from build123d import *

# Parameters (mm, degrees)
F0_W      = 24
F0_H      = 24
F0_R      = 2.6
F1_DEPTH  = 24
F2_SIZE   = 2
F4_DEPTH  = 8
F5_R      = 2
F7_DEPTH  = 8
F8_R      = 2
F9_SIZE   = 1.5
F10_R     = 1.75
F11_DEPTH = 25


with BuildPart() as f1:
    # F0 (on Top) → F1 (new body)
    with BuildSketch(Plane.XY):
        Rectangle(F0_W, F0_H)
        Circle(F0_R, mode=Mode.SUBTRACT)
    extrude(amount=F1_DEPTH)

    # F2
    f2_edges = [f1.edges().sort_by_distance(p)[0] for p in [
        (-12, -12, 12),
        (12, -12, 12),
        (-12, 12, 12),
        (12, 12, 12),
    ]]
    chamfer(f2_edges, length=F2_SIZE)

    # F3 (on Top) → F4 (cut)
    with BuildSketch(Plane.XY):
        with BuildLine():
            ThreePointArc((3.5, -6.5611658181), (6.3767557079, -3.8256873283), (7.4363228072, 0))
            ThreePointArc((7.4363228072, 0), (-3.8256873283, 6.3767557079), (-3.5, -6.5611658181))
            Line((-3.5, -6.5611658181), (-3.5, -3))
            Line((-3.5, -3), (3.5, -3))
            Line((3.5, -3), (3.5, -6.5611658181))
        make_face()
        with BuildLine():
            Line((-3.5, -3), (-3.5, -6.5611658181))
            ThreePointArc((-3.5, -6.5611658181), (0, -7.4363228072), (3.5, -6.5611658181))
            Line((3.5, -6.5611658181), (3.5, -3))
            Line((3.5, -3), (-3.5, -3))
        make_face()
        with BuildLine():
            ThreePointArc((3.5, -6.5611658181), (0, -7.4363228072), (-3.5, -6.5611658181))
            Line((-3.5, -6.5611658181), (-3.5, -13))
            Line((-3.5, -13), (3.5, -13))
            Line((3.5, -13), (3.5, -6.5611658181))
        make_face()
    extrude(amount=F4_DEPTH, mode=Mode.SUBTRACT)

    # F5
    f5_edges = [f1.edges().sort_by_distance(p)[0] for p in [
        (-3.5, -6.561166, 4),
        (3.5, -6.561166, 4),
    ]]
    fillet(f5_edges, radius=F5_R)

    # F6 (on face) → F7 (cut)
    with BuildSketch(Plane.XY.offset(24)):
        with BuildLine():
            ThreePointArc((3.5, -6.7461099902), (6.4946131525, -3.9471508712), (7.6, 0))
            ThreePointArc((7.6, 0), (-3.9471508712, 6.4946131525), (-3.5, -6.7461099902))
            Line((-3.5, -6.7461099902), (-3.5, -4.0145893581))
            Line((-3.5, -4.0145893581), (3.5, -4.0145893581))
            Line((3.5, -4.0145893581), (3.5, -6.7461099902))
        make_face()
        with BuildLine():
            Line((-3.5, -4.0145893581), (-3.5, -6.7461099902))
            ThreePointArc((-3.5, -6.7461099902), (0, -7.6), (3.5, -6.7461099902))
            Line((3.5, -6.7461099902), (3.5, -4.0145893581))
            Line((3.5, -4.0145893581), (-3.5, -4.0145893581))
        make_face()
        with BuildLine():
            ThreePointArc((3.5, -6.7461099902), (0, -7.6), (-3.5, -6.7461099902))
            Line((-3.5, -6.7461099902), (-3.5, -12))
            Line((-3.5, -12), (3.5, -12))
            Line((3.5, -12), (3.5, -6.7461099902))
        make_face()
    extrude(amount=-F7_DEPTH, mode=Mode.SUBTRACT)

    # F8
    f8_edges = [f1.edges().sort_by_distance(p)[0] for p in [
        (3.5, -6.74611, 20),
        (-3.5, -6.74611, 20),
    ]]
    fillet(f8_edges, radius=F8_R)

    # F9
    f9_edges = [f1.edges().sort_by_distance(p)[0] for p in [
        (3.5, -12, 20),
        (-3.5, -12, 20),
        (3.5, -12, 4),
        (-3.5, -12, 4),
    ]]
    chamfer(f9_edges, length=F9_SIZE)

    # F10 (on Top) → F11 (cut)
    with BuildSketch(Plane.XY):
        with Locations((-8.5, -8.5)):
            Circle(F10_R)
        with Locations((8.5, -8.5)):
            Circle(F10_R)
        with Locations((8.5, 8.5)):
            Circle(F10_R)
        with Locations((-8.5, 8.5)):
            Circle(F10_R)
    extrude(amount=F11_DEPTH, mode=Mode.SUBTRACT)


solid = f1.part
Verification items for the finished model (mm, model axes). A direction names the side the tool comes from. Coordinates: 2 decimals unless noted, no trailing zeros. Order: outer loops, then holes, each group sorted by start corner. A loop starts at its lowest first (then second) coordinate and runs counter-clockwise, first axis right, second up. Notation, with made-up numbers: M 49.25,32 L 96.25,32 A12 cw 96.25,49 Z; hole C -25,82 d10. An arc over 180 degrees is marked long. One line per item, written item: value. Start each with the question number.
Item 1: Scan lines: probe 1 along X at (y, z) = (-8.5, 7.5); probe 2 along Y at (x, z) = (8.5, 11). Record each from-to range of solid material in increasing order.
Item 2: Access from +Z, -Z, +X, -X, +Y, -Y to the whole of each face (thin tool, end or side, straight path). Record for faces 1 (the flat face through (3.5, -9, 4)), 2 (the flat face through (-11, 11, 12)), 3 (the flat face through (-4, -11, 20)), 4 (the cylindrical face through (3.7, -6.8, 4.1)).
Item 3: Sectioned sample at D-D (z = 14.75). Enter the section's corners in (x, y), then the cut area to 3 significant figures.
Item 4: Gauge pin test, flat ends, axial feed: pin 1 (7.5 mm diameter, centred on x = 0.5, y = -2.5, fed in from -Z); pin 2 (3 mm diameter, centred on x = 3, z = 18, fed in from -Y); pin 3 (6 mm diameter, centred on x = 0, y = 0, fed in from +Z). Record the tip position at first contact, or that the pin passes through.
Item 5: Sectioned sample at A-A (z = 21.5). Enter the section's corners in (x, y).
Item 6: Mould release check, pull along Y, two halves, no side actions. Record for faces 5 (the flat face through (-6, 6, 24)), 6 (the flat face through (11, 11, 12)), 7 (the cylindrical face through (-7.6, 10, 11.8)), 8 (the flat face through (4, -11, 4)): released by +Y, released by -Y, zero draft, split by the parting line, or undercut.
Item 7: Sectioned sample at B-B (x = 8.5). Enter the section's corners in (y, z), then the cut area to 3 significant figures.
Conclusion:
1. probe 1: x = -12 to -10.25, -6.75 to -3.5, 3.5 to 6.75, 10.25 to 12
1. probe 2: y = -12 to -10.25, -6.75 to 6.75, 10.25 to 12
2. face 1: -Z, -Y
2. face 2: +Z, -Z, -X, +Y
2. face 3: +Z, -Y
2. face 4: -Z
3. outline: M -12,-10 L -10,-12 L 10,-12 L 12,-10 L 12,10 L 10,12 L -10,12 L -12,10 Z; hole C -8.5,-8.5 d3.5; hole C -8.5,8.5 d3.5; hole C 0,0 d5.2; hole C 8.5,-8.5 d3.5; hole C 8.5,8.5 d3.5
3. area: 508 mm^2
4. pin 1: stops at z = 8
4. pin 2: stops at y = -11.5
4. pin 3: stops at z = 16
5. outline: M -12,-10 L -10,-12 L -5,-12 L -3.5,-10.5 L -3.5,-7.87 A2 ccw -4.35,-6.23 A7.6 cw long 4.35,-6.23 A2 ccw 3.5,-7.87 L 3.5,-10.5 L 5,-12 L 10,-12 L 12,-10 L 12,10 L 10,12 L -10,12 L -12,10 Z; hole C -8.5,-8.5 d3.5; hole C -8.5,8.5 d3.5; hole C 8.5,-8.5 d3.5; hole C 8.5,8.5 d3.5
6. face 5: zero draft
6. face 6: released by +Y
6. face 7: undercut
6. face 8: released by -Y
7. outline: M -12,0 L -10.25,0 L -10.25,24 L -12,24 Z; M -6.75,0 L 6.75,0 L 6.75,24 L -6.75,24 Z; M 10.25,0 L 12,0 L 12,24 L 10.25,24 Z
7. area: 408 mm^2
